Answer from the drawing. Dimensions are ordinates in mm from the lowest x, y and z of the part. Give positions to 0.01 mm unless a question says otherwise; leave off trailing zeros. Order: outer loops, then holes, each group sorted by start corner. A loop starts at its lowest first (then second) coordinate and runs counter-clockwise, first axis right, second up.
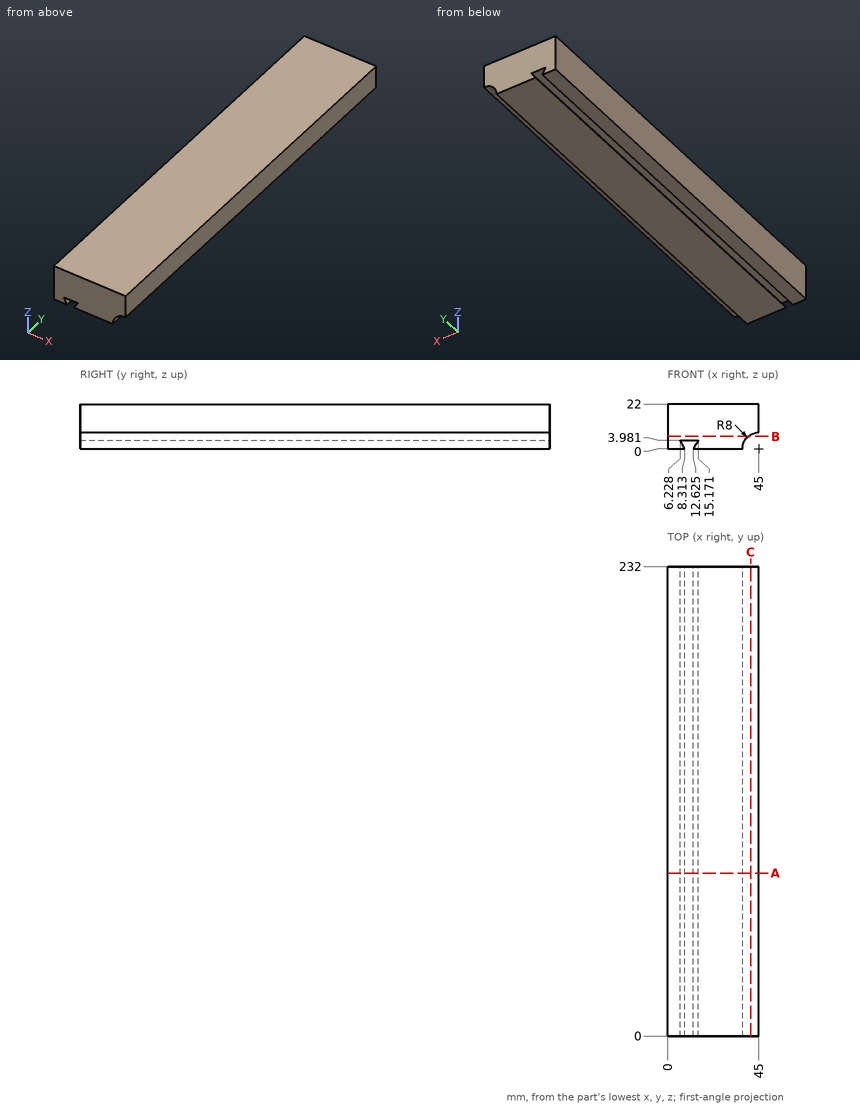
1) The part is cut by section A-A on y = 80.5. Determine the outline of the cut face in (x, z) (1 decimal), and give its area (3 significant figures).
Final values:
outline: (0, 0) - (8.3, 0) - (6.2, 4) - (15.2, 4) - (12.6, 0) - (37, 0) arc R8 cw to (45, 8) - (45, 22) - (0, 22) - close
area: 913 mm2
2) Consider L1, parallel to Z at x = 9.5, y = 185; L2, parallel to X at y = 94, z = 1.25 (1 decimal); L3, parallel to Z at x = 15, y = 30 (1 decimal). Determine where each line is inside the solid, lowest interval first.
Final values:
L1: z = 3.98 to 22
L2: x = 0 to 7.7, 13.4 to 37.1
L3: z = 0 to 3.7, 4 to 22
3) The part is cut by section C-C on x = 41. Determine the outline of the cut face in (y, z).
Final values:
outline: (0, 6.93) - (232, 6.93) - (232, 22) - (0, 22) - close
4) The part is cut by section B-B on z = 6. Determine the outline of the cut face in (x, y).
Final values:
outline: (0, 0) - (39.71, 0) - (39.71, 232) - (0, 232) - close
5) Given pin 1 (1.5 mm diameter, centred on y = 40.5, z = 5.5, fed in from +X) (1 decimal), flat-ended and moving along its own axis, determine where the tip first touches the part or whether it passes through.
Final values:
pin 1: stops at x = 40
